Read the model definition and answer for the solid it produces. Units are mm, in the model's axes. Coordinates: 2 decimals unless noted, no trailing zeros. Loops run counter-clockwise (first coordinate to the right, second up) from the corner with the lowest first, then second, coordinate; pieces in that order, holes last. Notation, with made-up numbers: (49, -23.5) - (87, -23.5) arc R33 ccw to (87, 14.5) - close; hole circle Ø6 at (-21.5, -37). An arc over 180 degrees is marked (long way). Use one line per item in the form item = value. Start each with the question number.
1) Consider line 1 (Z direction, x = 56.5, y = 15); line 2 (Z direction, x = 243, y = 18.5); line 3 (Y direction, x = 257.5, z = 9.5). Determine where each line is inside the solid, lowest interval first.
2) A cutting plane is placed at A-A (x = 179). Give the vertices of the cut face in (y, z).
3) A cutting plane is placed at B-B (y = 0). Give the vertices of the cut face in (x, z), and give its area (3 significant figures).
4) A cutting plane is placed at C-C (z = -7.5). Give the vertices of the cut face in (x, y).
5) Each of these flat-tipped pins is pushed along its axis until it touches: P1, Ø6, axis at x = 225.5, y = 3, coming from the +Z side; P2, Ø5, axis at x = 186, y = 2, coming from the -Z side; P3, Ø1, axis at x = 193.5, y = 8, coming from the -Z side. Where does it stop, or does it pass through?
from build123d import *

# Parameters (mm, degrees)
F1_DEPTH = 300


with BuildPart() as f1:
    # F0 (on Right) → F1 (new body)
    with BuildSketch(Plane.YZ):
        with BuildLine():
            ThreePointArc((-9, 28.618176), (-17.748239, -24.186773), (30, 0))
            ThreePointArc((30, 0), (24.186773, 17.748239), (9, 28.618176))
            Line((9, 28.618176), (9, 25))
            Line((9, 25), (0, 25))
            Line((0, 25), (-9, 25))
            Line((-9, 25), (-9, 28.618176))
        make_face()
    extrude(amount=F1_DEPTH)


solid = f1.part
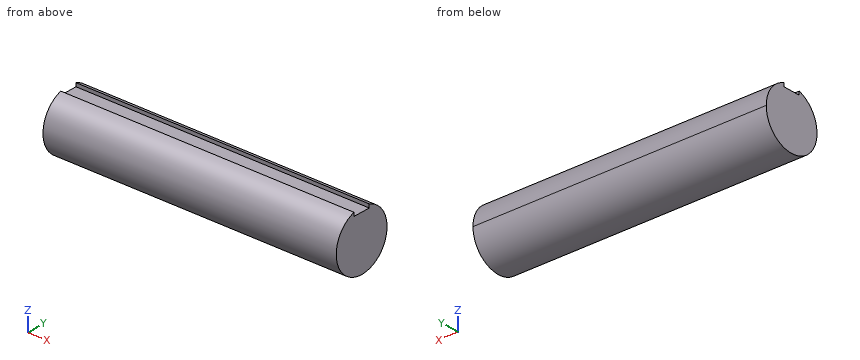
Found:
q1.line_1 = -25.98 to 25.98
q1.line_2 = -23.62 to 23.62
q1.line_3 = -28.46 to 28.46
q2.outline = (-9, 25) - (-9, 28.62) arc R30 ccw (long way) to (30, 0) arc R30 ccw to (9, 28.62) - (9, 25) - close
q3.outline = (0, -30) - (300, -30) - (300, 25) - (0, 25) - close
q3.area = 16,500 mm^2
q4.outline = (0, -29.05) - (300, -29.05) - (300, 29.05) - (0, 29.05) - close
q5.P1 = 25
q5.P2 = -30
q5.P3 = -29.05
